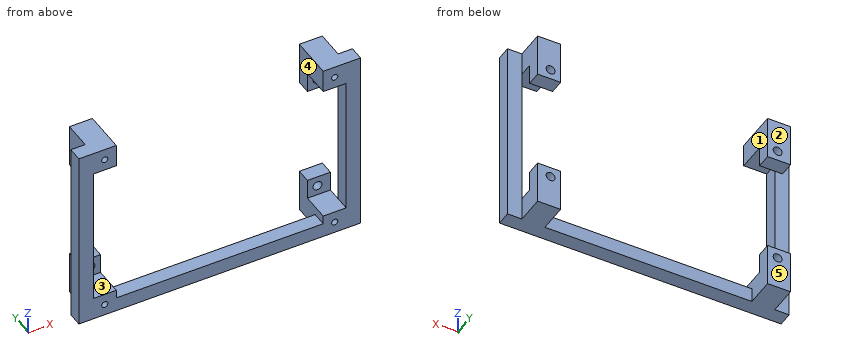
from build123d import *

# Parameters (mm, degrees)
SKETCH1_W             = 7
SKETCH1_H             = 7
BOSS_EXTRUDE1_DEPTH   = 5
BOSS_EXTRUDE1_2_DEPTH = 5
BOSS_EXTRUDE1_3_DEPTH = 5
BOSS_EXTRUDE1_4_DEPTH = 5
SKETCH2_R             = 1.55
CUT_EXTRUDE1_DEPTH    = 6
SKETCH4_W             = 8
SKETCH4_H             = 8
BOSS_EXTRUDE3_DEPTH   = 14.76
BOSS_EXTRUDE4_DEPTH   = 5
SKETCH6_R             = 1.0795
CUT_EXTRUDE2_DEPTH    = 10
SKETCH7_W             = 1
SKETCH7_H             = 7
BOSS_EXTRUDE5_DEPTH   = 5


with BuildPart() as part:
    # Sketch1 → Boss-Extrude1 (new body)
    with BuildSketch(Plane(origin=(0, 0, 0), x_dir=(1, 0, 0), z_dir=(0, 1, 0))):
        with Locations((-39.5, 21)):
            Rectangle(SKETCH1_W, SKETCH1_H)
    extrude(amount=BOSS_EXTRUDE1_DEPTH)


with BuildPart() as body_2:
    # Sketch1 → Boss-Extrude1 2 (new body)
    with BuildSketch(Plane(origin=(0, 0, 0), x_dir=(1, 0, 0), z_dir=(0, 1, 0))):
        with Locations((39.5, 21)):
            Rectangle(SKETCH1_W, SKETCH1_H)
    extrude(amount=BOSS_EXTRUDE1_2_DEPTH)


with BuildPart() as body_3:
    # Sketch1 → Boss-Extrude1 3 (new body)
    with BuildSketch(Plane(origin=(0, 0, 0), x_dir=(1, 0, 0), z_dir=(0, 1, 0))):
        with Locations((-39.5, -21)):
            Rectangle(SKETCH1_W, SKETCH1_H)
    extrude(amount=BOSS_EXTRUDE1_3_DEPTH)


with BuildPart() as body_4:
    # Sketch1 → Boss-Extrude1 4 (new body)
    with BuildSketch(Plane(origin=(0, 0, 0), x_dir=(1, 0, 0), z_dir=(0, 1, 0))):
        with Locations((39.5, -21)):
            Rectangle(SKETCH1_W, SKETCH1_H)
    extrude(amount=BOSS_EXTRUDE1_4_DEPTH)


with BuildPart() as cut_extrude1_tool:
    # Sketch2 → Cut-Extrude1 (new body, through all)
    with BuildSketch(Plane(origin=(0, 5, 0), x_dir=(1, 0, 0), z_dir=(0, 1, 0))):
        with Locations((-39.5, 21)):
            Circle(SKETCH2_R)
        with Locations((39.5, 21)):
            Circle(SKETCH2_R)
        with Locations((39.5, -21)):
            Circle(SKETCH2_R)
        with Locations((-39.5, -21)):
            Circle(SKETCH2_R)
    extrude(amount=-CUT_EXTRUDE1_DEPTH)


with BuildPart() as part_1:
    add(part.part)

    # Cut-Extrude1: cut by cut_extrude1_tool
    add(cut_extrude1_tool.part, mode=Mode.SUBTRACT)



with BuildPart() as body_2_1:
    add(body_2.part)

    # Cut-Extrude1: cut by cut_extrude1_tool
    add(cut_extrude1_tool.part, mode=Mode.SUBTRACT)


with BuildPart() as body_3_1:
    add(body_3.part)

    # Cut-Extrude1: cut by cut_extrude1_tool
    add(cut_extrude1_tool.part, mode=Mode.SUBTRACT)


with BuildPart() as body_4_1:
    add(body_4.part)

    # Cut-Extrude1: cut by cut_extrude1_tool
    add(cut_extrude1_tool.part, mode=Mode.SUBTRACT)


with BuildPart() as part_2:
    add(part_1.part)

    add(body_2_1.part)  # Boss-Extrude3 merges body 2

    add(body_3_1.part)  # Boss-Extrude3 merges body 3

    add(body_4_1.part)  # Boss-Extrude3 merges body 4
    # Sketch4 → Boss-Extrude3 (add)
    with BuildSketch(Plane(origin=(0, 5, 0), x_dir=(1, 0, 0), z_dir=(0, 1, 0))):
        with Locations((40, 28.5)):
            Rectangle(SKETCH4_W, SKETCH4_H)
        with Locations((40, -28.5)):
            Rectangle(SKETCH4_W, SKETCH4_H)
        with Locations((-40, -28.5)):
            Rectangle(SKETCH4_W, SKETCH4_H)
        with Locations((-40, 28.5)):
            Rectangle(SKETCH4_W, SKETCH4_H)
    extrude(amount=-BOSS_EXTRUDE3_DEPTH)

    # Sketch5 → Boss-Extrude4 (add)
    with BuildSketch(Plane.XZ.offset(9.76)):
        Polygon((-49, 32.5), (-49, -32.5), (49, -32.5), (49, 32.5), (44, 32.5), (44, -27.5), (-44, -27.5), (-44, 32.5), align=None)
    extrude(amount=-BOSS_EXTRUDE4_DEPTH)

    # Sketch6 → Cut-Extrude2 (cut)
    with BuildSketch(Plane(origin=(0, -4.76, 0), x_dir=(-1, 0, 0), z_dir=(0, 1, 0))):
        with Locations((40, 28.5)):
            Circle(SKETCH6_R)
        with Locations((40, -28.5)):
            Circle(SKETCH6_R)
        with Locations((-40, -28.5)):
            Circle(SKETCH6_R)
        with Locations((-40, 28.5)):
            Circle(SKETCH6_R)
    extrude(amount=-CUT_EXTRUDE2_DEPTH, mode=Mode.SUBTRACT)

    # Sketch7 → Boss-Extrude5 (add)
    with BuildSketch(Plane(origin=(0, 5, 0), x_dir=(1, 0, 0), z_dir=(0, 1, 0))):
        with Locations((43.5, -21)):
            Rectangle(SKETCH7_W, SKETCH7_H)
        with Locations((43.5, 21)):
            Rectangle(SKETCH7_W, SKETCH7_H)
        with Locations((-43.5, 21)):
            Rectangle(SKETCH7_W, SKETCH7_H)
        with Locations((-43.5, -21)):
            Rectangle(SKETCH7_W, SKETCH7_H)
    extrude(amount=-BOSS_EXTRUDE5_DEPTH)


solid = part_2.part
Read the model definition and answer for the solid it produces. Units are mm, in the model's axes. Face numbers are marked on the shaded views. A direction names the side the tool comes from. Coordinates: 2 decimals unless noted, no trailing zeros. Loops run counter-clockwise (first coordinate to the right, second up) from the corner with the lowest first, then second, coordinate; pieces in that order, holes last.
Q1. The mould has two halves that part along X. Classify the marked faces 1 and 2: +X half, -X half, draft (parallel to the pull), parting line (faces both ways), or undercut.
Q2. The part is cut by section A-A on y = 2. Write down the section's boundary in (x, z).
Q3. Consider probe 1 along X at (y, z) = (2.9, -21); probe 2 along Z at (x, y) = (40, -8.65); probe 3 along Z at (x, y) = (-39.5, 2.55). Determine where each line is inside the solid, lowest interval first.
Q4. The part is cut by section D-D on z = 18.5. Write down the section's boundary in (x, y), and give its area (3 significant figures).
Q5. Each of these flat-tipped pins is pushed along its axis until it touches: pin 1 Ø4 at (x, z) = (-39.5, -21) entering from -Y; pin 2 Ø2.5 at (x, z) = (-39.5, 21) entering from -Y; pin 3 Ø4 at (x, z) = (-46.5, -8) entering from +Y; pin 4 Ø3 at (x, y) = (0.5, -7) entering from +Z. Where does it stop, or does it pass through?
Q6. Which of the six approach directions +Z, -Z, +X, -X, +Y, -Y give full straight-line access (tool end or side, diameter ignored) to the marked faces 3, 4 and 5?
Q7. The part is cut by section B-B on z = 2.5. Write down the section's boundary in (x, y).
Q8. The part is cut by section C-C on z = -21. Write down the section's boundary in (x, y).
Results below:
1. face 1: undercut
1. face 2: draft
2. outline: (-44, -32.5) - (-36, -32.5) - (-36, -17.5) - (-44, -17.5) - close; (-44, 17.5) - (-36, 17.5) - (-36, 32.5) - (-44, 32.5) - close; (36, -32.5) - (44, -32.5) - (44, -17.5) - (36, -17.5) - close; (36, 17.5) - (44, 17.5) - (44, 32.5) - (36, 32.5) - close; hole circle Ø3.1 at (-39.5, -21); hole circle Ø3.1 at (-39.5, 21); hole circle Ø3.1 at (39.5, -21); hole circle Ø3.1 at (39.5, 21)
3. probe 1: x = -44 to -41.05, -37.95 to -36, 36 to 37.95, 41.05 to 44
3. probe 2: z = -32.5 to -29.58, -27.42 to -24.5, 24.5 to 27.42, 29.58 to 32.5
3. probe 3: z = -32.5 to -22.55, -19.45 to -17.5, 17.5 to 19.45, 22.55 to 32.5
4. outline: (-49, -9.76) - (-44, -9.76) - (-44, -4.76) - (-49, -4.76) - close; (-44, 0) - (-36, 0) - (-36, 5) - (-44, 5) - close; (36, 0) - (44, 0) - (44, 5) - (36, 5) - close; (44, -9.76) - (49, -9.76) - (49, -4.76) - (44, -4.76) - close
4. area: 130 mm2
5. pin 1: stops at y = 0
5. pin 2: passes through
5. pin 3: stops at y = -4.76
5. pin 4: stops at z = -27.5
6. face 3: -Y
6. face 4: +Z, +Y, -Y
6. face 5: +Z, -Z, +X, -X, +Y
7. outline: (-49, -9.76) - (-44, -9.76) - (-44, -4.76) - (-49, -4.76) - close; (44, -9.76) - (49, -9.76) - (49, -4.76) - (44, -4.76) - close
8. outline: (-49, -9.76) - (-44, -9.76) - (-44, -4.76) - (-49, -4.76) - close; (-44, 0) - (-41.05, 0) - (-41.05, 5) - (-44, 5) - close; (-37.95, 0) - (-36, 0) - (-36, 5) - (-37.95, 5) - close; (36, 0) - (37.95, 0) - (37.95, 5) - (36, 5) - close; (41.05, 0) - (44, 0) - (44, 5) - (41.05, 5) - close; (44, -9.76) - (49, -9.76) - (49, -4.76) - (44, -4.76) - close
